Autodesk Inventor part; units mm, degrees
ref_plane "YZ Plane" through (0, 0, 0) normal (1, 0, 0) x (0, 1, 0)
ref_plane "XZ Plane" through (0, 0, 0) normal (0, 1, 0) x (-1, 0, 0)
ref_plane "XY Plane" through (0, 0, 0) normal (0, 0, 1) x (1, 0, 0)
sketch "Sketch1" plane through (0, 0, 0) normal (0, 1, 0) x (-1, 0, 0)
  circle A0 centre (-19.704, -123.7953) radius 1.5
  circle A1 centre (-26.6684, -112.9171) radius 1.5
  circle A2 centre (-75.7396, -112.9171) radius 1.5
  line L0 (-101.204, -106.1137) -> (-89.704, -106.1137)
  line L1 (-101.204, -106.1137) -> (-66.204, -106.1137)
  arc A3 (-101.204, -112.9171) -> (-1.204, -151.1137) centre (-1.204, -1.1137) ccw
  line L2 (-101.204, -106.1137) -> (-101.204, -112.9171)
  line L3 (-89.704, -106.1137) -> (-78.204, -106.1137)
  circle A4 centre (17.296, 121.5679) radius 1.5
  circle A5 centre (17.296, 84.5679) radius 1.5
  line L4 (63.796, 103.8863) -> (63.796, 66.8863)
  circle A6 centre (24.2604, 110.6897) radius 1.5
  circle A7 centre (73.3316, 110.6897) radius 1.5
  line L5 (98.796, 103.8863) -> (63.796, 103.8863)
  arc A8 (98.796, 110.6897) -> (-1.204, 148.8863) centre (-1.204, -1.1137) ccw
  line L6 (75.796, 43.8863) -> (87.296, 43.8863)
  circle A9 centre (73.3316, 37.0829) radius 1.5
  line L7 (87.296, 43.8863) -> (98.796, 43.8863)
  circle A10 centre (-19.704, 121.5679) radius 1.5
  circle A11 centre (-1.204, 148.8863) radius 1.5
  circle A12 centre (-26.6684, 110.6897) radius 1.5
  circle A13 centre (-75.7396, 110.6897) radius 1.5
  line L8 (-101.204, 103.8863) -> (-66.204, 103.8863)
  line L9 (-101.204, 103.8863) -> (-101.204, 110.6897)
  arc A14 (-1.204, 148.8863) -> (-101.204, 110.6897) centre (-1.204, -1.1137) ccw
  line L10 (-2.704, 148.8863) -> (-1.204, 148.8863)
  line L11 (0.296, 148.8863) -> (-1.204, 148.8863)
  line L12 (63.796, -69.1137) -> (60.796, -69.1137)
  line L13 (38.396, -69.1137) -> (41.396, -69.1137)
  line L14 (63.796, -46.1137) -> (98.796, -46.1137)
  line L15 (60.796, -69.1137) -> (60.796, -57.6137)
  line L16 (41.396, -69.1137) -> (41.396, -57.6137)
  line L17 (63.796, -46.1137) -> (60.796, -46.1137)
  line L18 (60.796, -46.1137) -> (60.796, -57.6137)
  line L19 (41.396, -46.1137) -> (41.396, -57.6137)
  line L20 (38.396, -46.1137) -> (41.396, -46.1137)
  line L21 (38.396, -57.6137) -> (38.396, -46.1137)
  circle A15 centre (73.3316, -39.3103) radius 1.5
  line L22 (38.396, -57.6137) -> (38.396, -69.1137)
  circle A16 centre (17.296, -123.7953) radius 1.5
  circle A17 centre (17.296, -86.7953) radius 1.5
  circle A18 centre (15.296, -60.7953) radius 1.5
  line L23 (75.796, -106.1137) -> (87.296, -106.1137)
  line L24 (87.296, -106.1137) -> (98.796, -106.1137)
  circle A19 centre (24.2604, -112.9171) radius 1.5
  line L25 (63.796, -106.1137) -> (63.796, -69.1137)
  circle A20 centre (73.3316, -112.9171) radius 1.5
  arc A21 (-1.204, -151.1137) -> (98.796, -112.9171) centre (-1.204, -1.1137) ccw
  line L26 (98.796, -106.1137) -> (63.796, -106.1137)
  circle A22 centre (-17.704, 34.2047) radius 1.5
  line L27 (-101.204, 43.8863) -> (-89.704, 43.8863)
  line L28 (-89.704, 43.8863) -> (-78.204, 43.8863)
  circle A23 centre (-75.7396, 37.0829) radius 1.5
  circle A24 centre (-75.7396, -39.3103) radius 1.5
  line L29 (-66.204, -46.1137) -> (-101.204, -46.1137)
  line L30 (-66.204, 43.8863) -> (-101.204, 43.8863)
  line L31 (-66.204, -46.1137) -> (-63.204, -46.1137)
  line L32 (-101.204, -1.1137) -> (-101.204, -46.1137)
  line L33 (-101.204, -1.1137) -> (-101.204, 43.8863)
  line L34 (98.796, -1.1137) -> (98.796, -46.1137)
  line L35 (98.796, -1.1137) -> (98.796, -46.1137)
  line L36 (98.796, -1.1137) -> (98.796, 43.8863)
  line L37 (98.796, -1.1137) -> (98.796, 43.8863)
  circle A25 centre (-19.704, 84.5679) radius 1.5
  line L38 (-66.204, 103.8863) -> (-66.204, 66.8863)
  line L39 (-40.804, 66.8863) -> (-43.804, 66.8863)
  line L40 (-40.804, 55.3863) -> (-40.804, 66.8863)
  line L41 (-43.804, 66.8863) -> (-43.804, 55.3863)
  line L42 (-66.204, 66.8863) -> (-63.204, 66.8863)
  line L43 (-63.204, 66.8863) -> (-63.204, 55.3863)
  line L44 (-40.804, 55.3863) -> (-40.804, 43.8863)
  line L45 (-40.804, 43.8863) -> (-43.804, 43.8863)
  line L46 (-43.804, 43.8863) -> (-43.804, 55.3863)
  line L47 (-63.204, 43.8863) -> (-63.204, 55.3863)
  line L48 (-66.204, 43.8863) -> (-63.204, 43.8863)
  circle A26 centre (-19.704, -86.7953) radius 1.5
  line L49 (-66.204, -106.1137) -> (-66.204, -69.1137)
  line L50 (-66.204, -69.1137) -> (-63.204, -69.1137)
  line L51 (-40.804, -69.1137) -> (-43.804, -69.1137)
  line L52 (-43.804, -69.1137) -> (-43.804, -57.6137)
  line L53 (-40.804, -57.6137) -> (-40.804, -69.1137)
  line L54 (-63.204, -46.1137) -> (-63.204, -57.6137)
  circle A27 centre (-17.704, -60.7953) radius 1.5
  line L55 (-43.804, -46.1137) -> (-43.804, -57.6137)
  line L56 (-40.804, -46.1137) -> (-43.804, -46.1137)
  line L57 (-40.804, -57.6137) -> (-40.804, -46.1137)
  line L58 (-63.204, -69.1137) -> (-63.204, -57.6137)
  line L59 (98.796, 103.8863) -> (98.796, 110.6897)
  line L60 (98.796, 103.8863) -> (98.796, 110.6897)
  line L61 (98.796, -106.1137) -> (98.796, -112.9171)
  line L62 (98.796, -106.1137) -> (98.796, -112.9171)
  line L63 (63.796, 43.8863) -> (98.796, 43.8863)
  line L64 (63.796, 66.8863) -> (60.796, 66.8863)
  line L65 (38.396, 66.8863) -> (41.396, 66.8863)
  line L66 (60.796, 66.8863) -> (60.796, 55.3863)
  line L67 (41.396, 66.8863) -> (41.396, 55.3863)
  line L68 (38.396, 55.3863) -> (38.396, 66.8863)
  line L69 (63.796, 43.8863) -> (60.796, 43.8863)
  line L70 (60.796, 43.8863) -> (60.796, 55.3863)
  line L71 (41.396, 43.8863) -> (41.396, 55.3863)
  line L72 (38.396, 43.8863) -> (41.396, 43.8863)
  line L73 (38.396, 55.3863) -> (38.396, 43.8863)
  circle A28 centre (15.296, 34.2047) radius 1.5
  point P0 (0, 0)
  point P1 (0.296, 148.8863)
  point P2 (-2.704, 148.8788)
extrude "Extrusion1" add sketch "Sketch1" along normal blind 3 contours L0 L1 L49 L50 L58 L54 L31 L29 L32 L33 L27 L28 L30 L48 L47 L43 L42 L38 L8 L9 A14 A11 A8 L59 L5 L4 L64 L66 L70 L69 L63 L6 L7 L36 L34 L14 L17 L18 L15 L12 L25 L26 L23 L24 L61 A21 A3 L2
properties part number "ChasisInferior"
Input: part model. Units: mm. Frame: model coordinates. Give positions to 0.01 mm unless a question says otherwise; leave off trailing zeros. Write each loop counter-clockwise with the first axis right and the second up, starting at its lowest first coordinate (ties: lowest second). Pieces come first, ordered by that corner, then holes. Notation, with made-up numbers: (23, 43) - (40, 43) arc R23 ccw to (40, 79) - close; hole circle Ø2 at (2.25, -14). An arc over 180 degrees is marked (long way). Write item = value, one per line. Start each with the question number.
1) Cut plane C-C (z = 92). Return loops of the section in (x, y).
2) Pin query (flat end, axial travel): pin 1 (3.5 mm diameter, centred on x = 17.7, z = -60.8, fed in from -Y); pin 2 (0.9 mm diameter, centred on y = 1, z = 59, fed in from -X); pin 3 (0.9 mm diameter, centred on y = 1.5, z = -87, fed in from +X); pin 4 (0.9 mm diameter, centred on x = -63, y = 1.5, fed in from -Z). Return the tip coordinate at first contact, or that it passes through.
3) Material intervals for L1, parallel to X at y = 2.75, z = 55; L2, parallel to Z at x = -78.5, y = 1.85; L3, parallel to Z at x = 88.5, y = 2.7, sorted ascending. Write a range as [from, to].
4) Cut plane D-D (y = 1.75). Give the number of separate pieces and of enclosed holes in the cut face, and give its area (3 significant figures).
5) Cut plane A-A (z = 52.5). Return loops of the section in (x, y), and give its area (3 significant figures).
6) Cut plane B-B (x = -79). Return loops of the section in (y, z), and give its area (3 significant figures).
Answers follow:
q1.outline = (-63.8, 0) - (66.2, 0) - (66.2, 3) - (-63.8, 3) - close
q2.pin_1 = 0
q2.pin_2 = -60.8
q2.pin_3 = 66.2
q2.pin_4 = -136.89
q3.L1 = [-60.8, -41.4], [-38.4, 40.8], [43.8, 63.2]
q3.L2 = [-128.19, -106.11], [-46.11, 43.89], [103.89, 125.96]
q3.L3 = [-123.09, -106.11], [-46.11, 43.89], [103.89, 120.87]
q4.separate_pieces = 1
q4.enclosed_holes = 28
q4.area = 46,100 mm^2
q5.outline = (-60.8, 0) - (-41.4, 0) - (-41.4, 3) - (-60.8, 3) - close; (-38.4, 0) - (40.8, 0) - (40.8, 3) - (-38.4, 3) - close; (43.8, 0) - (63.2, 0) - (63.2, 3) - (43.8, 3) - close
q5.area = 354 mm^2
q6.outline = (0, -127.87) - (3, -127.87) - (3, -106.11) - (0, -106.11) - close; (0, -46.11) - (3, -46.11) - (3, 43.89) - (0, 43.89) - close; (0, 103.89) - (3, 103.89) - (3, 125.64) - (0, 125.64) - close
q6.area = 401 mm^2
